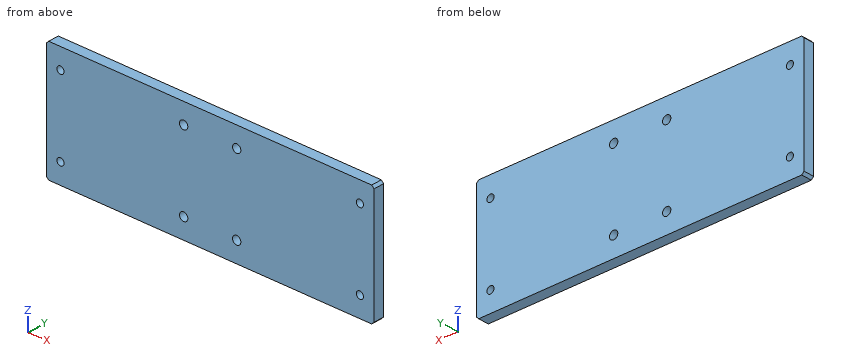
from build123d import *

# Parameters (mm, degrees)
F0_W     = 277
F0_H     = 100
F0_R     = 3
F0_R_2   = 3.5
F1_DEPTH = 9
F2_SIZE  = 2
F3_SIZE  = 2
F4_SIZE  = 2
F5_SIZE  = 2


with BuildPart() as f1:
    # F0 (on Front) → F1 (new body)
    with BuildSketch(Plane.XZ):
        with Locations((138.5, 50)):
            Rectangle(F0_W, F0_H)
        with Locations((12, 17)):
            Circle(F0_R, mode=Mode.SUBTRACT)
        with Locations((116.098186, 17)):
            Circle(F0_R_2, mode=Mode.SUBTRACT)
        with Locations((160.901814, 17)):
            Circle(F0_R_2, mode=Mode.SUBTRACT)
        with Locations((265, 17)):
            Circle(F0_R, mode=Mode.SUBTRACT)
        with Locations((12, 83)):
            Circle(F0_R, mode=Mode.SUBTRACT)
        with Locations((116.098186, 83)):
            Circle(F0_R_2, mode=Mode.SUBTRACT)
        with Locations((160.901814, 83)):
            Circle(F0_R_2, mode=Mode.SUBTRACT)
        with Locations((265, 83)):
            Circle(F0_R, mode=Mode.SUBTRACT)
    extrude(amount=F1_DEPTH)

    # F2
    f2_edges = [f1.edges().sort_by_distance(p)[0] for p in [
        (277, -4.5, 100),
    ]]
    chamfer(f2_edges, length=F2_SIZE)

    # F3
    f3_edges = [f1.edges().sort_by_distance(p)[0] for p in [
        (277, -4.5, 0),
    ]]
    chamfer(f3_edges, length=F3_SIZE)

    # F4
    f4_edges = [f1.edges().sort_by_distance(p)[0] for p in [
        (0, -4.5, 0),
    ]]
    chamfer(f4_edges, length=F4_SIZE)

    # F5
    f5_edges = [f1.edges().sort_by_distance(p)[0] for p in [
        (0, -4.5, 100),
    ]]
    chamfer(f5_edges, length=F5_SIZE)


solid = f1.part
Geometry check sheet. Reference: the model listing, model coordinates, mm. Give positions to 0.01 mm unless a question says otherwise; leave off trailing zeros. Write each loop counter-clockwise with the first axis right and the second up, starting at its lowest first coordinate (ties: lowest second). Pieces come first, ordered by that corner, then holes.
1) Go/stop test with flat-tipped pins: pin 1 Ø4 at (x, z) = (116.1, 17) entering from -Y; pin 2 Ø10 at (x, z) = (84, 82.5) entering from +Y. Record where each tip stops, or that it passes through.
Values follow:
pin 1: passes through
pin 2: stops at y = 0
2) Cross-section at A-A (z = 17). Record the boundary of the cut face in (x, y).
Values follow:
outline: (0, -9) - (9, -9) - (9, 0) - (0, 0) - close; (15, -9) - (112.6, -9) - (112.6, 0) - (15, 0) - close; (119.6, -9) - (157.4, -9) - (157.4, 0) - (119.6, 0) - close; (164.4, -9) - (262, -9) - (262, 0) - (164.4, 0) - close; (268, -9) - (277, -9) - (277, 0) - (268, 0) - close
3) Cross-section at B-B (x = 265). Record the boundary of the cut face in (y, z), plus the area to 3 significant figures.
Values follow:
outline: (-9, 0) - (0, 0) - (0, 14) - (-9, 14) - close; (-9, 20) - (0, 20) - (0, 80) - (-9, 80) - close; (-9, 86) - (0, 86) - (0, 100) - (-9, 100) - close
area: 792 mm2
4) Thickness scan on line 1 (Z direction, x = 12, y = -4.25); line 2 (X direction, y = -1.75, z = 15.5); line 3 (Z direction, x = 13, y = -8.25). Record the ranges inside material, lowest first.
Values follow:
line 1: z = 0 to 14, 20 to 80, 86 to 100
line 2: x = 0 to 9.4, 14.6 to 112.94, 119.26 to 157.74, 164.06 to 262.4, 267.6 to 277
line 3: z = 0 to 14.17, 19.83 to 80.17, 85.83 to 100
